Verification items for this drawing (mm, ordinates from the low corner). A direction names the side the tool comes from. Round coordinates to 2 decimals unless told otherwise and drop trailing zeros. Loops run counter-clockwise (first coordinate to the right, second up) from the corner with the lowest first, then second, coordinate; pieces in that order, holes last. Notation, with made-up numbers: (86, -14.5) - (128, -14.5) arc R16 ccw to (128, 10.5) - close; hole circle Ø2 at (-14, 21.5). An arc over 180 degrees is marked (long way). Write item = value, one per line.
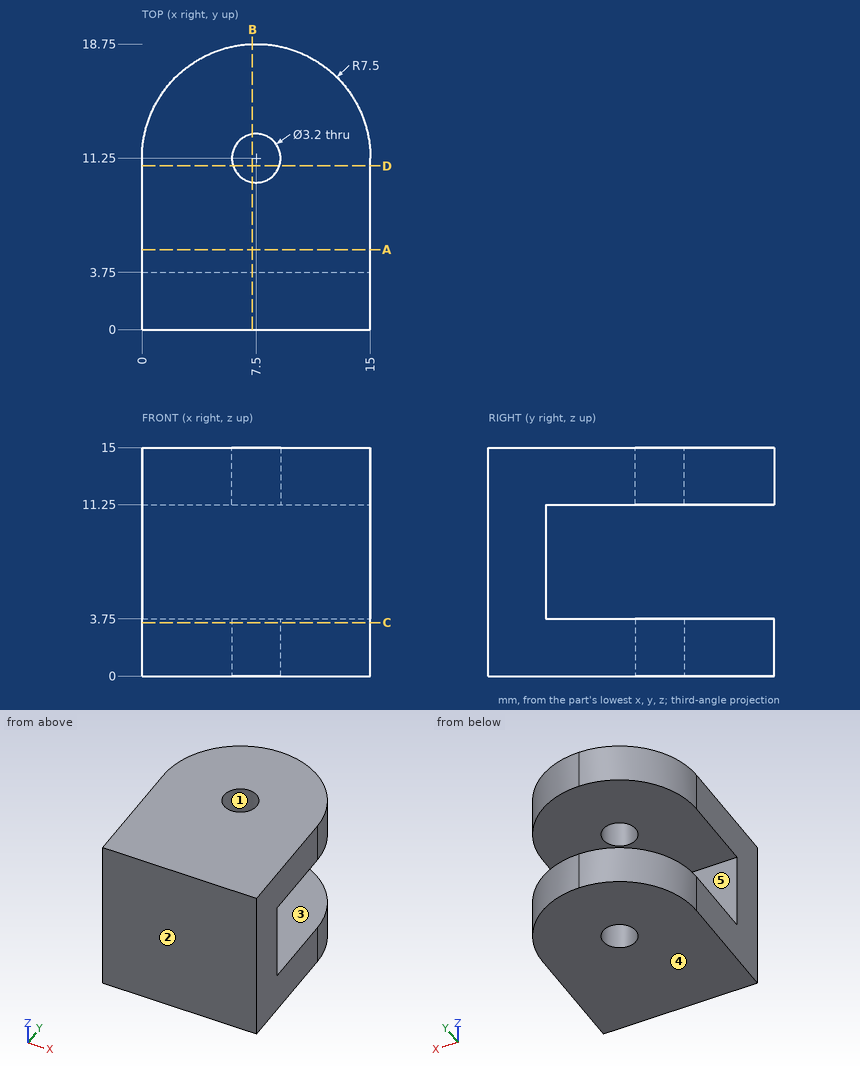
(1) Section check D-D (y = 10.75). Enter the section's corners in (x, z).
Answers follow:
outline = (0, 0) - (5.98, 0) - (5.98, 3.75) - (0, 3.75) - close; (0, 11.25) - (5.98, 11.25) - (5.98, 15) - (0, 15) - close; (9.02, 0) - (15, 0) - (15, 3.75) - (9.02, 3.75) - close; (9.02, 11.25) - (15, 11.25) - (15, 15) - (9.02, 15) - close
(2) Section check C-C (z = 3.5). Enter the section's corners in (x, y), then the cut area to 3 significant figures.
Answers follow:
outline = (0, 0) - (15, 0) - (15, 11.25) arc R7.5 ccw to (0, 11.25) - close; hole circle Ø3.2 at (7.5, 11.25)
area = 249 mm²
(3) Mould release check, pull along Y, two halves, no side actions. Record for the marked faces 1, 2 and 3: pulls with the +Y half, pulls with the -Y half, needs draft (parallel to the pull), parting line crosses it, or undercut.
Answers follow:
face_1 = undercut
face_2 = pulls with the -Y half
face_3 = needs draft
(4) Scan lines: L1, parallel to Z at x = 11.75, y = 7.5; L2, parallel to Y at x = 7.5, z = 1.15; L3, parallel to Y at x = 14, z = 10.5. Record each from-to range of solid material in increasing order. Write a range as [from, to].
Answers follow:
L1 = [0, 3.75], [11.25, 15]
L2 = [0, 9.65], [12.85, 18.75]
L3 = [0, 3.75]
(5) Section check A-A (y = 5.25). Enter the section's corners in (x, z), then the cut area to 4 significant figures.
Answers follow:
outline = (0, 0) - (15, 0) - (15, 3.75) - (0, 3.75) - close; (0, 11.25) - (15, 11.25) - (15, 15) - (0, 15) - close
area = 112.5 mm²
(6) Section check B-B (x = 7.25). Enter the section's corners in (y, z), then the cut area to 3 significant figures.
Answers follow:
outline = (0, 0) - (9.67, 0) - (9.67, 3.75) - (3.75, 3.75) - (3.75, 11.25) - (9.67, 11.25) - (9.67, 15) - (0, 15) - close; (12.83, 0) - (18.75, 0) - (18.75, 3.75) - (12.83, 3.75) - close; (12.83, 11.25) - (18.75, 11.25) - (18.75, 15) - (12.83, 15) - close
area = 145 mm²
(7) Set-up check for the marked faces 4 and 5: record each of +Z, -Z, +X, -X, +Y, -Y from which the full face is reachable in a straight line by a thin tool's end or side.
Answers follow:
face_4 = -Z, +X, -X, +Y, -Y
face_5 = +X, -X, +Y
(8) Gauge pin test, flat ends, axial feed: pin 1 (5 mm diameter, centred on y = 10.5, z = 8, fed in from +X); pin 2 (2 mm diameter, centred on x = 11, z = 6, fed in from +Y). Record the tip position at first contact, or that the pin passes through.
Answers follow:
pin_1 = through
pin_2 = 3.75
